```python
from build123d import *

# Parameters (mm, degrees)
BOX_W             = 100
BOX_H             = 5
BOX_DEPTH         = 27
PAD_DEPTH         = 2.5
CYLINDER_R        = 12.5
CYLINDER_DEPTH    = 72
BOX001_W          = 104
BOX001_H          = 7
BOX001_DEPTH      = 27
PAD001_DEPTH      = 3.5
CYLINDER001_R     = 15.5
CYLINDER001_DEPTH = 75


with BuildPart() as tip_hole:
    # Box → Box (new body)
    with BuildSketch(Plane(origin=(-50, -2.5, 62.5), x_dir=(1, 0, 0), z_dir=(0, 0, 1))):
        with Locations((50, 2.5)):
            Rectangle(BOX_W, BOX_H)
    extrude(amount=BOX_DEPTH)


with BuildPart() as internal_duct:
    # Sketch → Pad (new body, symmetric)
    with BuildSketch(Plane(origin=(-68, 0, -12.5), x_dir=(1, 0, 0), z_dir=(0, -1, 0))):
        Polygon((55.48275, 0), (17.98275, 75), (117.98275, 75), (80.48275, 0), align=None)
    extrude(amount=PAD_DEPTH, both=True)


with BuildPart() as holes:
    # Cylinder → Cylinder (new body)
    with BuildSketch(Plane.XY.offset(-15.5)):
        Circle(CYLINDER_R)
    extrude(amount=CYLINDER_DEPTH)

    # Fusion: union tip hole, internal duct
    add(tip_hole.part)
    add(internal_duct.part)


with BuildPart() as tip_body:
    # Box001 → Box001 (new body)
    with BuildSketch(Plane(origin=(-52, -3.5, 62.5), x_dir=(1, 0, 0), z_dir=(0, 0, 1))):
        with Locations((52, 3.5)):
            Rectangle(BOX001_W, BOX001_H)
    extrude(amount=BOX001_DEPTH)


with BuildPart() as internal_duct_wall:
    # Sketch001 → Pad001 (new body, symmetric)
    with BuildSketch(Plane(origin=(-65.5, 0, -12.5), x_dir=(1, 0, 0), z_dir=(0, -1, 0))):
        Polygon((49.929678, 0), (13.429678, 75), (117.429678, 75), (80.929678, 0), align=None)
    extrude(amount=PAD001_DEPTH, both=True)


with BuildPart() as body_with_holes:
    # Cylinder001 → Cylinder001 (new body)
    with BuildSketch(Plane.XY.offset(-12.5)):
        Circle(CYLINDER001_R)
    extrude(amount=CYLINDER001_DEPTH)

    # Fusion001: union tip body, internal duct wall
    add(tip_body.part)
    add(internal_duct_wall.part)

    # Cut: cut Holes
    add(holes.part, mode=Mode.SUBTRACT)


solid = body_with_holes.part
```
The model under review builds one solid part; all positions refer to its coordinate system, in mm. A direction names the side the tool comes from. Round coordinates to 2 decimals unless told otherwise and drop trailing zeros. Order: outer loops, then holes, each group sorted by start corner. A loop starts at its lowest first (then second) coordinate and runs counter-clockwise, first axis right, second up.
(1) Wall thickness on L1, parallel to Y at x = 17.5, z = 72.5; L2, parallel to X at y = 2, z = 76; L3, parallel to Y at x = 0, z = 30.5: over which ranges is each line inside the solid? List them lowest first.
Working result:
L1: y = -3.5 to -2.5, 2.5 to 3.5
L2: x = -52 to -50, 50 to 52
L3: y = -15.5 to -12.5, 12.5 to 15.5
(2) Take a section at A-A, the plane x = -1. State the section outline as (y, z) points, plus the area to 3 significant figures.
Working result:
outline: (-15.47, -12.5) - (-12.46, -12.5) - (-12.46, 56.5) - (-2.5, 56.5) - (-2.5, 89.5) - (-3.5, 89.5) - (-3.5, 62.5) - (-15.47, 62.5) - close; (2.5, 56.5) - (12.46, 56.5) - (12.46, -12.5) - (15.47, -12.5) - (15.47, 62.5) - (3.5, 62.5) - (3.5, 89.5) - (2.5, 89.5) - close
area: 625 mm2
(3) Take a section at D-D, the plane x = 30.5. State the section outline as (y, z) points.
Working result:
outline: (-3.5, 18.47) - (3.5, 18.47) - (3.5, 89.5) - (2.5, 89.5) - (2.5, 23.53) - (-2.5, 23.53) - (-2.5, 89.5) - (-3.5, 89.5) - close
(4) Mouldability with a two-part tool opening along Y and no side actions: class faces 4 (the face through (0.291, 15.497, 24.475)), 5 (the face through (50, 0, 76)), 6 (the face through (-0.291, -15.497, 24.475)), 7 (the face through (-4, -3, 89.5)) as released by +Y, released by -Y, zero draft, split by the parting line, or undercut.
Working result:
face 4: released by +Y
face 5: undercut
face 6: released by -Y
face 7: zero draft
(5) Tool access review of faces 1 (the face through (-50, 0, 76)), 2 (the face through (0, 6, 56.5)), 3 (the face through (0, 8, 62.5)): name each direction out of +Z, -Z, +X, -X, +Y, -Y from which nothing blocks a thin tool from reaching the whole face with its end or side.
Working result:
face 1: +Z
face 2: -Z
face 3: +Z, +X, -X, +Y
(6) For P1, Ø1, axis at y = 4.5, z = 18.5, coming from the -X side (3 decimals); P2, Ø8, axis at x = -1, y = -1.5, coming from the -Z side; P3, Ø1.5, axis at y = -1, z = 75.5, coming from the -X side, all flat-tipped, find the tip position at first contact; note any pin that passes through.
Working result:
P1: stops at x = -14.975
P2: stops at z = 56.5
P3: stops at x = -52
(7) Take a section at C-C, the plane y = 11. State the section outline as (x, z) points.
Working result:
outline: (-10.92, -12.5) - (-5.94, -12.5) - (-5.94, 56.5) - (5.94, 56.5) - (5.94, -12.5) - (10.92, -12.5) - (10.92, 62.5) - (-10.92, 62.5) - close
(8) Take a section at B-B, the plane z = 44. State the section outline as (x, y) points, plus the area to 3 significant figures.
Working result:
outline: (-43.07, -3.5) - (-15.1, -3.5) arc R15.5 ccw to (15.1, -3.5) - (42.93, -3.5) - (42.93, 3.5) - (15.1, 3.5) arc R15.5 ccw to (-15.1, 3.5) - (-43.07, 3.5) - close; hole (-40.77, -2.5) - (-12.25, -2.5) arc R12.5 ccw to (12.25, -2.5) - (40.73, -2.5) - (40.73, 2.5) - (12.25, 2.5) arc R12.5 ccw to (-12.25, 2.5) - (-40.77, 2.5) - close
area: 367 mm2
